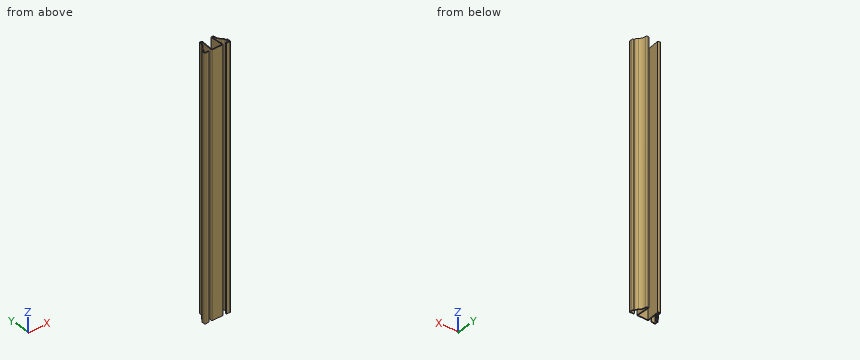
from build123d import *

# Parameters (mm, degrees)
EXTRUDE_THIN1_DEPTH = 285.75
FILLET1_R           = 0.889


with BuildPart() as part:
    # Sketch1 → Extrude-Thin1 (new body)
    with BuildSketch(Plane.XY):
        with BuildLine():
            Line((9.525, 0.396875), (14.2875, 0))
            Line((14.2875, 0), (14.2875, 4.7625))
            Line((14.2875, 4.7625), (12.7, 4.7625))
            ThreePointArc((12.7, 4.7625), (12.221883718, 6.842274605), (10.883532847, 8.504464286))
            ThreePointArc((10.883532847, 8.504464286), (8.423051877, 11.795038582), (7.9375, 15.875))
            Line((7.9375, 15.875), (4.7625, 15.875))
            Line((4.7625, 15.875), (5.55625, 1.285875))
            Line((5.55625, 1.285875), (-5.55625, 1.285875))
            Line((-5.55625, 1.285875), (-4.7625, 15.875))
            Line((-4.7625, 15.875), (-7.9375, 15.875))
            ThreePointArc((-7.9375, 15.875), (-8.423051877, 11.795038582), (-10.883532847, 8.504464286))
            ThreePointArc((-10.883532847, 8.504464286), (-12.221883718, 6.842274605), (-12.7, 4.7625))
            Line((-12.7, 4.7625), (-14.2875, 4.7625))
            Line((-14.2875, 4.7625), (-14.2875, 0))
            Line((-14.2875, 0), (-9.525, 0.396875))
            Line((-9.525, 0.396875), (-9.598827432, 1.282804179))
            Line((-9.598827432, 1.282804179), (-13.3985, 0.966164798))
            Line((-13.3985, 0.966164798), (-13.3985, 3.8735))
            Line((-13.3985, 3.8735), (-11.707603613, 3.8735))
            ThreePointArc((-11.707603613, 3.8735), (-11.594220702, 6.040152518), (-10.333606715, 7.805964286))
            ThreePointArc((-10.333606715, 7.805964286), (-7.800475833, 10.997107398), (-6.970486535, 14.986))
            Line((-6.970486535, 14.986), (-5.701182591, 14.986))
            Line((-5.701182591, 14.986), (-6.494932591, 0.396875))
            Line((-6.494932591, 0.396875), (6.494932591, 0.396875))
            Line((6.494932591, 0.396875), (5.701182591, 14.986))
            Line((5.701182591, 14.986), (6.970486535, 14.986))
            ThreePointArc((6.970486535, 14.986), (7.800475833, 10.997107398), (10.333606715, 7.805964286))
            ThreePointArc((10.333606715, 7.805964286), (11.594220702, 6.040152518), (11.707603613, 3.8735))
            Line((11.707603613, 3.8735), (13.3985, 3.8735))
            Line((13.3985, 3.8735), (13.3985, 0.966164798))
            Line((13.3985, 0.966164798), (9.598827432, 1.282804179))
            Line((9.598827432, 1.282804179), (9.525, 0.396875))
        make_face()
    extrude(amount=-EXTRUDE_THIN1_DEPTH)

    # Fillet1
    fillet1_edges = [part.edges().sort_by_distance(p)[0] for p in [
        (11.707603613, 3.8735, -142.875),
        (6.494932591, 0.396875, -142.875),
        (-6.494932591, 0.396875, -142.875),
        (-11.707603613, 3.8735, -142.875),
        (-14.2875, 0, -142.875),
        (-14.2875, 4.7625, -142.875),
        (-7.9375, 15.875, -142.875),
        (-4.7625, 15.875, -142.875),
        (4.7625, 15.875, -142.875),
        (7.9375, 15.875, -142.875),
        (14.2875, 4.7625, -142.875),
        (14.2875, 0, -142.875),
    ]]
    fillet(fillet1_edges, radius=FILLET1_R)


solid = part.part
Can you work these out from the model? Positions are in its coordinate system, mm. Give positions to 0.01 mm unless a question says otherwise; leave off trailing zeros. Order: outer loops, then holes, each group sorted by start corner. A loop starts at its lowest first (then second) coordinate and runs counter-clockwise, first axis right, second up. Notation, with made-up numbers: M 24,-20.5 L 53,-20.5 A27 cw 53,-3.5 Z; hole C 34.25,65 d10. An arc over 180 degrees is marked long. Use one line per item in the form item = value. Start each with the question number.
Item 1: If I drill on line 1 along X through (y, z) = (11.75, -263); line 2 along X through (y, z) = (13.5, -44.5); line 3 along Y through (x, z) = (-0.5, -134), over which ranges is the centre line in solid material (lowest first)?
Item 2: Will these pins go through, and if not, where does the flat tip stop? pin 1 Ø1 at (x, z) = (-6.5, -169) entering from -Y; pin 2 Ø12 at (x, z) = (2.5, -168) entering from -Y; pin 3 Ø3.5 at (x, z) = (-2, -178) entering from +Y.
Item 3: If we section it at A-A (y = 11.75): Write out the boundary of the cut face in (x, z).
Outcome:
q1.line_1 = -8.44 to -7.49, -5.88 to -4.99, 4.99 to 5.88, 7.49 to 8.44
q1.line_2 = -7.95 to -7.05, -5.78 to -4.89, 4.89 to 5.78, 7.05 to 7.95
q1.line_3 = 0.4 to 1.29
q2.pin_1 = 0.52
q2.pin_2 = 0.4
q2.pin_3 = 1.29
q3.outline = M -8.44,-285.75 L -7.49,-285.75 L -7.49,0 L -8.44,0 Z; M -5.88,-285.75 L -4.99,-285.75 L -4.99,0 L -5.88,0 Z; M 4.99,-285.75 L 5.88,-285.75 L 5.88,0 L 4.99,0 Z; M 7.49,-285.75 L 8.44,-285.75 L 8.44,0 L 7.49,0 Z
